The drawing under review shows one solid part. Ordinate dimensions are in mm from its lowest x, y, z. A direction names the side the tool comes from. Round coordinates to 2 decimals unless told otherwise and drop trailing zeros. Loops run counter-clockwise (first coordinate to the right, second up) from the corner with the lowest first, then second, coordinate; pieces in that order, holes last. Notation, with made-up numbers: (-4.75, -40) -> (48.25, -40) arc R30 cw to (48.25, -5) -> close; hole circle Ø2 at (48, 60.25). An arc over 180 degrees is marked (long way). Answer as CSV lines item,"result". Start each with the question number.
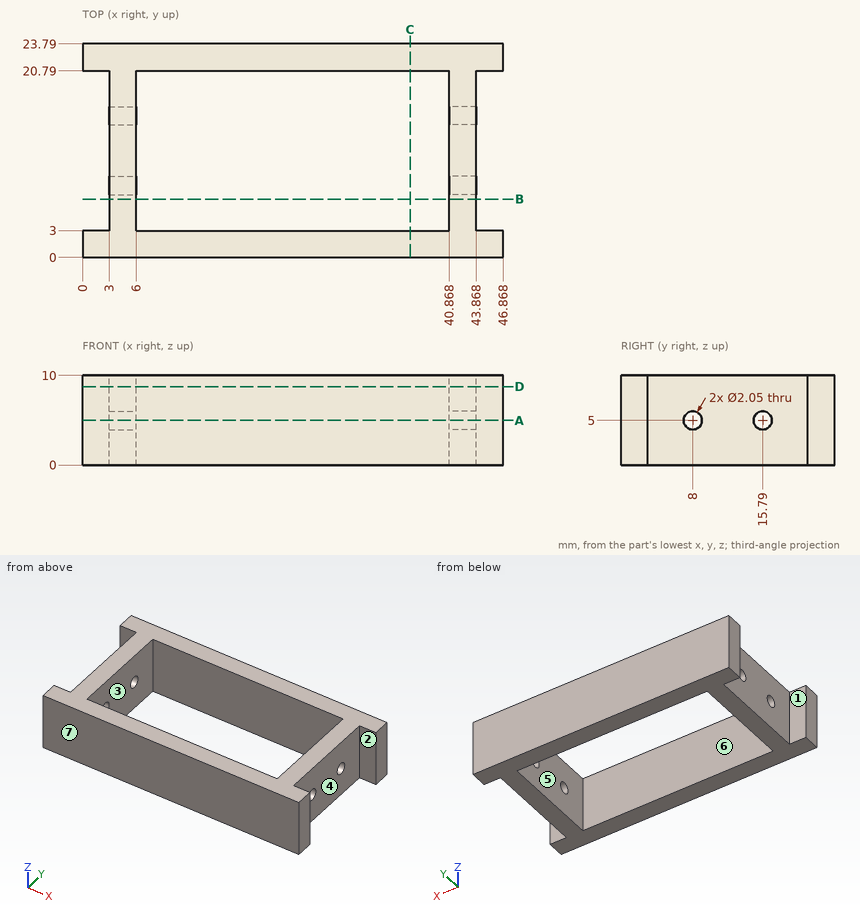
Q1. Add section B-B, the plane y = 6.5. Give the boundary of the cut face in (x, z), and give its area (3 significant figures).
Q2. Add section A-A, the plane z = 5. State how many separate pieces and enclosed holes the cut face has, and give its area (3 significant figures).
Q3. To check wall thickness, follow probe 1 along Y at (x, z) = (17.5, 8.75); probe 2 along X at (y, z) = (17, 4.5); probe 3 along Y at (x, z) = (41.8, 5) (3 decimals). State the ranges of each line that lie inside material, in increasing order. Write a range as from..to.
Q4. Machinability: for the marked faces 1, 2 and 3, which of the approach directions +Z, -Z, +X, -X, +Y, -Y give a long, thin tool a straight path to every point of the face, cutting with its end or side? Answer none if there is none.
Q5. For pin 1 Ø3 at (y, z) = (8.5, 2.5) entering from -X; pin 2 Ø5 at (y, z) = (9.5, 5.5) entering from +X, all flat-tipped, find the tip position at first contact; note any pin that passes through.
Q6. Add section D-D, the plane z = 8.75. Give the boundary of the cut face in (x, y).
Q7. Add section C-C, the plane x = 36.5. Give the boundary of the cut face in (y, z), and give its area (3 significant figures).
Q8. Mouldability with a two-part tool opening along X and no side actions: class the marked faces 4, 5, 6 and 7 as pulls with the +X half, pulls with the -X half, needs draft (parallel to the pull), parting line crosses it, or undercut.
Worked answers:
1,outline,"(3, 0) -> (6, 0) -> (6, 10) -> (3, 10) -> close; (40.87, 0) -> (43.87, 0) -> (43.87, 10) -> (40.87, 10) -> close"
1,area,"60.0 mm^2"
2,separate pieces,"4"
2,enclosed holes,"0"
2,area,"363 mm^2"
3,probe 1,"y = 0..3, 20.79..23.79"
3,probe 2,"x = 3..6, 40.87..43.87"
3,probe 3,"y = 0..6.975, 9.025..14.765, 16.815..23.79"
4,face 1,"+Z, -Z, -X"
4,face 2,"+Z, -Z, +X"
4,face 3,"+Z, -Z"
5,pin 1,"stops at x = 3"
5,pin 2,"stops at x = 43.87"
6,outline,"(0, 0) -> (46.87, 0) -> (46.87, 3) -> (43.87, 3) -> (43.87, 20.79) -> (46.87, 20.79) -> (46.87, 23.79) -> (0, 23.79) -> (0, 20.79) -> (3, 20.79) -> (3, 3) -> (0, 3) -> close; hole (6, 3) -> (40.87, 3) -> (40.87, 20.79) -> (6, 20.79) -> close"
7,outline,"(0, 0) -> (3, 0) -> (3, 10) -> (0, 10) -> close; (20.79, 0) -> (23.79, 0) -> (23.79, 10) -> (20.79, 10) -> close"
7,area,"60.0 mm^2"
8,face 4,"pulls with the +X half"
8,face 5,"undercut"
8,face 6,"undercut"
8,face 7,"needs draft"
